from build123d import *

# Parameters (mm, degrees)
SKETCH_1_W          = 100
SKETCH_1_H          = 100
EXTRUDE_1_DEPTH     = 3
SKETCH_2_R          = 1.65
CUT_EXTRUDE_1_DEPTH = 3
FILLET_1_R          = 2
FILLET_2_R          = 2


with BuildPart() as part:
    # 草图1 → 凸台-拉伸1 (new body)
    with BuildSketch(Plane(origin=(0, 0, 0), x_dir=(0, 0, -1), z_dir=(1, 0, 0))):
        with Locations((50, -50)):
            Rectangle(SKETCH_1_W, SKETCH_1_H)
    extrude(amount=EXTRUDE_1_DEPTH)

    # 草图2 → 切除-拉伸1 (cut)
    with BuildSketch(Plane(origin=(3, 0, 0), x_dir=(0, 0, -1), z_dir=(1, 0, 0))):
        with Locations((3.5, -3.5)):
            Circle(SKETCH_2_R)
        with Locations(Location((96.5, -3.5, 0), (0, 0, 180))):
            Circle(SKETCH_2_R)
        with Locations((96.5, -96.5)):
            Circle(SKETCH_2_R)
        with Locations(Location((3.5, -96.5, 0), (0, 0, 180))):
            Circle(SKETCH_2_R)
    extrude(amount=-CUT_EXTRUDE_1_DEPTH, mode=Mode.SUBTRACT)

    # 圆角1
    fillet_1_edges = [part.edges().sort_by_distance(p)[0] for p in [
        (1.5, 0, -100),
    ]]
    fillet(fillet_1_edges, radius=FILLET_1_R)

    # 圆角2
    fillet_2_edges = [part.edges().sort_by_distance(p)[0] for p in [
        (1.5, 0, 0),
        (1.5, -100, -100),
        (1.5, -100, 0),
    ]]
    fillet(fillet_2_edges, radius=FILLET_2_R)


solid = part.part
Geometry check sheet. Reference: the model listing, model coordinates, mm. Round coordinates to 2 decimals unless told otherwise and drop trailing zeros. Loops run counter-clockwise (first coordinate to the right, second up) from the corner with the lowest first, then second, coordinate; pieces in that order, holes last.
Item 1: Cross-section at A-A on z = -96.5. Record the boundary of the cut face in (x, y).
Item 2: Thickness scan on line 1 (Y direction, x = 1.8, z = -3.5); line 2 (Z direction, x = 1.55, y = -4.5). Record the ranges inside material, lowest first.
Item 3: Gauge pin test, flat end, axial feed: pin 1 (2 mm diameter, centred on y = -96.5, z = -3.5, fed in from +X). Record the tip position at first contact, or that the pin passes through.
Item 4: Mould release check, pull along Y, two halves, no side actions. Record for faces 1 (the flat face through (1, -100, -49)), 2 (the flat face through (0, -49, -49)), 3 (the cylindrical face through (1.52, -97.5, -95.19)): pulls with the +Y half, pulls with the -Y half, needs draft (parallel to the pull), parting line crosses it, or undercut.
Answer sheet:
1. outline: (0, -100) - (3, -100) - (3, -98.15) - (0, -98.15) - close; (0, -94.85) - (3, -94.85) - (3, -5.15) - (0, -5.15) - close; (0, -1.85) - (3, -1.85) - (3, 0) - (0, 0) - close
2. line 1: y = -100 to -98.15, -94.85 to -5.15, -1.85 to 0
2. line 2: z = -100 to -97.81, -95.19 to -4.81, -2.19 to 0
3. pin 1: passes through
4. face 1: pulls with the -Y half
4. face 2: needs draft
4. face 3: undercut
